from build123d import *

# Parameters (mm, degrees)
F0_W      = 49.6500022709
F0_H      = 49.5000034571
F1_DEPTH  = 50
F2_W      = 25
F2_H      = 25
F3_DEPTH  = 25
F4_R      = 17.6184560371
F5_DEPTH  = 25
F7_DEPTH  = 25
F8_DEPTH  = 25
F9_DEPTH  = 55
F10_DEPTH = 55
F11_DEPTH = 100
F13_DEPTH = 25


with BuildPart() as f1:
    # F0 (on Top) → F1 (new body)
    with BuildSketch(Plane.XY):
        with Locations((24.8250011355, 24.7500017285)):
            Rectangle(F0_W, F0_H)
    extrude(amount=F1_DEPTH)

    # F2 (on face) → F3 (join)
    with BuildSketch(Plane.XZ):
        with Locations((23.4000021592, 24.4588267358)):
            Rectangle(F2_W, F2_H)
    extrude(amount=F3_DEPTH)

    # F4 (on face) → F5 (join)
    with BuildSketch(Plane.XY.offset(50)):
        with Locations((20.5500014126, 25.5000013858)):
            Circle(F4_R)
    extrude(amount=F5_DEPTH)

    # F6 (on face) → F7 (join)
    with BuildSketch(Plane.YZ.offset(49.6500022709)):
        Polygon((23.6848843281, 29.1616055147), (24.3537883277, 26.5821856483), (25.6675029629, 24.2637824769), (27.5365007525, 22.3643913453), (29.8334125856, 21.0134526203), (32.4017077168, 20.3030305434), (35.066361077, 20.2815392052), (37.6457809434, 20.9504432048), (39.9641841148, 22.26415784), (41.8635752464, 24.1331556296), (43.2145139714, 26.4300674627), (43.9249360483, 28.9983625938), (43.9464273865, 31.6630159541), (43.2775233869, 34.2424358205), (41.9638087517, 36.5608389919), (40.0948109622, 38.4602301235), (37.797899129, 39.8111688485), (35.2296039979, 40.5215909253), (32.5649506376, 40.5430822636), (29.9855307712, 39.874178264), (27.6671275998, 38.5604636288), (25.7677364683, 36.6914658392), (24.4167977433, 34.3945540061), (23.7063756664, 31.826258875), align=None)
    extrude(amount=F7_DEPTH)

    # F8 (add): a face of the model
    f8_faces = [f1.faces().sort_by_distance(p)[0] for p in [
        (74.6500022709, 33.8156558573, 30.4123107344),
    ]]
    extrude(f8_faces, amount=F8_DEPTH)

    # F9 (cut): a face of the model
    f9_faces = [f1.faces().sort_by_distance(p)[0] for p in [
        (99.6500022709, 33.8156558573, 30.4123107344),
    ]]
    extrude(f9_faces, amount=-F9_DEPTH, mode=Mode.SUBTRACT)

    # F10 (add): a face of the model
    f10_faces = [f1.faces().sort_by_distance(p)[0] for p in [
        (44.6500022709, 33.8156558573, 30.4123107344),
    ]]
    extrude(f10_faces, amount=F10_DEPTH)

    # F11 (cut): a face of the model
    f11_faces = [f1.faces().sort_by_distance(p)[0] for p in [
        (99.6500022709, 33.8156558573, 30.4123107344),
    ]]
    extrude(f11_faces, amount=-F11_DEPTH, mode=Mode.SUBTRACT)

    # F12 (on face) → F13 (join)
    with BuildSketch(Plane.XZ.offset(25)):
        with BuildLine():
            Line((35.9000021592, 11.9588267358), (35.9000021592, 20.0868558522))
            ThreePointArc((35.9000021592, 20.0868558522), (23.4000021592, 26.8690533376), (10.9000021592, 20.0868558522))
            Line((10.9000021592, 20.0868558522), (10.9000021592, 11.9588267358))
            Line((10.9000021592, 11.9588267358), (35.9000021592, 11.9588267358))
        make_face()
    extrude(amount=F13_DEPTH)


solid = f1.part
The model under review builds one solid part; all positions refer to its coordinate system, in mm. A direction names the side the tool comes from. Round coordinates to 2 decimals unless told otherwise and drop trailing zeros. Loops run counter-clockwise (first coordinate to the right, second up) from the corner with the lowest first, then second, coordinate; pieces in that order, holes last. Notation, with made-up numbers: M 10.25,82 L 55.25,82 A29 ccw 55.25,107 Z; hole C 10,3 d3. An arc over 180 degrees is marked long. Answer as CSV lines item,"result". Start each with the question number.
Item 1: Consider section A-A (x = 45). Write out the cut boundary in (y, z).
Item 2: Consider section C-C (y = 14.5). Write out the cut boundary in (x, z), then the cut area to 3 significant figures.
Item 3: For faces 1 (the face through (23.608, -37.325, 26.868)), 2 (the face through (36, 14, 50)), 3 (the face through (25.173, 43.617, 32.935)), 4 (the face through (20, 26, 75)), list the 3-axis set-ups (+Z, -Z, +X, -X, +Y, -Y) from which the entire face can be reached by the end or side of a thin tool; tool diameter is ignored.
Item 4: Wall thickness on line 1 (Y direction, x = 27.5, z = 26.5); line 2 (Y direction, x = 4.5, z = 42); line 3 (Z direction, x = 33.5, y = -15.5): over which ranges is each line inside the solid? List them lowest first. Write a range as [from, to].
Item 5: Mouldability with a two-part tool opening along Y and no side actions: class faces 5 (the face through (23, -25, 11.959)), 6 (the face through (25.17, 25.1, 35.56)), 7 (the face through (23, -50, 18)), 8 (the face through (25.173, 24.067, 33.128)) as released by +Y, released by -Y, zero draft, split by the parting line, or undercut.
Item 6: Insertion check: P1, Ø12, axis at x = 11.5, z = 66.5, coming from the +Y side; P2, Ø20, axis at y = -15.5, z = 30.5, coming from the -X side; P3, Ø6, axis at x = 16.5, y = -27, coming from the -Z side. Each pin has a flat end and moves straight along its axis. Give the tip position at first contact, or say it passes through.
Item 7: Consider section B-B (z = 19). Write out the cut boundary in (x, y).
Answer:
1,outline,"M 0,0 L 49.5,0 L 49.5,50 L 0,50 Z; hole M 23.68,29.16 L 24.35,26.58 L 25.67,24.26 L 27.54,22.36 L 29.83,21.01 L 32.4,20.3 L 35.07,20.28 L 37.65,20.95 L 39.96,22.26 L 41.86,24.13 L 43.21,26.43 L 43.92,29 L 43.95,31.66 L 43.28,34.24 L 41.96,36.56 L 40.09,38.46 L 37.8,39.81 L 35.23,40.52 L 32.56,40.54 L 29.99,39.87 L 27.67,38.56 L 25.77,36.69 L 24.42,34.39 L 23.71,31.83 Z"
2,outline,"M 0,0 L 49.65,0 L 49.65,50 L 34.31,50 L 34.31,75 L 6.79,75 L 6.79,50 L 0,50 Z"
2,area,"3,170 mm^2"
3,face 1,"+Z, -Y"
3,face 2,"+Z"
3,face 3,"+X, -X"
3,face 4,"+Z, +X, -X, +Y, -Y"
4,line 1,"y = [-25, 24.4], [43.23, 49.5]"
4,line 2,"y = [0, 49.5]"
4,line 3,"z = [11.96, 36.96]"
5,face 5,"zero draft"
5,face 6,"undercut"
5,face 7,"released by -Y"
5,face 8,"undercut"
6,P1,"stops at y = 42.85"
6,P2,"stops at x = 10.9"
6,P3,"stops at z = 11.96"
7,outline,"M 0,0 L 10.9,0 L 10.9,-50 L 35.9,-50 L 35.9,0 L 49.65,0 L 49.65,49.5 L 0,49.5 Z"
